```python
from build123d import *

# Parameters (mm, degrees)
SKETCH1_R                 = 2.5
BOSS_EXTRUDE1_DEPTH       = 12
F_3_CLEARANCE_HOLE1_D     = 2.794
F_3_CLEARANCE_HOLE1_DEPTH = 5
F_3_CLEARANCE_HOLE1_TIP   = 0.839402285
SKETCH4_W                 = 0.4
SKETCH4_H                 = 0.12


with BuildPart() as part:
    # Sketch1 → Boss-Extrude1 (new, symmetric)
    with BuildSketch(Plane(origin=(0, 0, 0), x_dir=(0, 0, -1), z_dir=(1, 0, 0))):
        Circle(SKETCH1_R)
    extrude(amount=BOSS_EXTRUDE1_DEPTH, both=True)

    # #3 Clearance Hole1
    with Locations(Plane.ZY.offset(12)):
        with Locations((0, 0)):
            Hole(F_3_CLEARANCE_HOLE1_D / 2, depth=F_3_CLEARANCE_HOLE1_DEPTH)
            with Locations((0, 0, -(F_3_CLEARANCE_HOLE1_DEPTH + F_3_CLEARANCE_HOLE1_TIP / 2))):  # 118° drill point
                Cone(0, F_3_CLEARANCE_HOLE1_D / 2, F_3_CLEARANCE_HOLE1_TIP, mode=Mode.SUBTRACT)

    # Sketch4 → Cut-Revolve1 (revolve, cut)
    with BuildSketch(Plane(origin=(0, 0, 0), x_dir=(1, 0, 0), z_dir=(0, 1, 0))):
        with Locations((10.6, 2.44)):
            Rectangle(SKETCH4_W, SKETCH4_H)
        with Locations((8.8, 2.44)):
            Rectangle(SKETCH4_W, SKETCH4_H)
        with Locations((-2.8, 2.44)):
            Rectangle(SKETCH4_W, SKETCH4_H)
        with Locations((-4.6, 2.44)):
            Rectangle(SKETCH4_W, SKETCH4_H)
        with Locations((1.8, 2.44)):
            Rectangle(SKETCH4_W, SKETCH4_H)
        with Locations((4.2, 2.44)):
            Rectangle(SKETCH4_W, SKETCH4_H)
    revolve(axis=Axis((13.2, 0, 0), (-1, 0, 0)), mode=Mode.SUBTRACT)


solid = part.part
```
For this review, take the finished solid that the model builds, in its own axes (mm). Round coordinates to 2 decimals unless told otherwise and drop trailing zeros. Write each loop counter-clockwise with the first axis right and the second up, starting at its lowest first coordinate (ties: lowest second). Pieces come first, ordered by that corner, then holes. Notation, with made-up numbers: (-13.5, -29) -> (-2.5, -29) arc R21 ccw to (-2.5, -21) -> close; hole circle Ø8 at (6.25, 31). An arc over 180 degrees is marked (long way). Use one line per item in the form item = value.
1) Clearance check with flat-ended pins moving along their axes: pin 1 (1.5 mm diameter, centred on y = -0.5, z = 0, fed in from -X); pin 2 (1 mm diameter, centred on x = 8.5, z = -1, fed in from -Y); pin 3 (1.5 mm diameter, centred on x = -4, y = -1.5, fed in from +Z). State where each tip first meets the part, or that it passes through.
Found:
pin_1 = -6.91
pin_2 = -2.45
pin_3 = 2.38
2) To check wall thickness, follow L1, parallel to Y at x = -8.55, z = 0; L2, parallel to Z at x = -9.5, y = -1.15. State the ranges of each line that lie inside material, in increasing order. Write a range as from..to.
Found:
L1 = -2.5..-1.4, 1.4..2.5
L2 = -2.22..-0.79, 0.79..2.22
3) Take a section at A-A, the plane x = -3.5. Write out the cut boundary in (y, z).
Found:
outline = circle Ø5 at (0, 0)
4) Mouldability with a two-part tool opening along Z and no side actions: class faces 1 (the flat face through (-12, -1.1, -1.1)), 2 (the cylindrical face through (-9.46, -0.85, 1.11)), 3 (the cylindrical face through (4.203, 2.323, 0.516)) as +Z half, -Z half, draft (parallel to the pull), parting line (faces both ways), or undercut.
Found:
face_1 = draft
face_2 = undercut
face_3 = parting line
